Here's how the part is built. I have some questions about the finished solid (model axes, mm). Face numbers are marked on the shaded views. A direction names the side the tool comes from. Coordinates: 2 decimals unless noted, no trailing zeros. Write each loop counter-clockwise with the first axis right and the second up, starting at its lowest first coordinate (ties: lowest second). Pieces come first, ordered by that corner, then holes. Notation, with made-up numbers: (-32, 14) -> (-26, 14) arc R19 ccw to (-26, 43) -> close; hole circle Ø3 at (66, 55). An arc over 180 degrees is marked (long way). Answer in a Markdown table with one row per item. Add a question column.
Autodesk Fusion 360 part; units mm, degrees
sketch "Sketch1" plane through (0, 0, 0) normal (0, 1, 0) x (1, 0, 0)
  line L0 (-6.9583, -4.2531) -> (7.1417, -4.2531)
  line L1 (7.1417, -4.2531) -> (7.1417, 4.7469)
  line L2 (7.1417, 4.7469) -> (-6.9583, 4.7469)
  line L3 (-6.9583, 4.7469) -> (-6.9583, -4.2531)
  line L4 (-6.9583, -4.2531) -> (-2.4583, -4.2531)
  line L5 (-2.4583, -4.2531) -> (-2.4583, 4.7469)
  line L6 (-2.4583, 4.7469) -> (-6.9583, 4.7469)
  line L7 (-6.9583, 4.7469) -> (-6.9583, -4.2531)
  dimension "d4" = 14.1
  dimension "d5" = 9
  dimension "d7" = 4.5
  dimension "d8" = 9
extrude "Extrude1" add sketch "Sketch1" along normal blind 15.4 contours L0 L2 L3 L4 L5 L6 L7
extrude "Extrude2" add sketch "Sketch1" along normal blind 3 contours L0 L1 L2 L5
sketch "Sketch2" plane through (-2.4583, 0, 0) normal (1, 0, 0) x (0, 1, 0)
  line L0 (3, 4.2531) -> (3, -4.7469)
  line L1 (3, -4.7469) -> (15.4, -4.7469)
  line L2 (15.4, -4.7469) -> (15.4, 4.2531)
  line L3 (15.4, 4.2531) -> (3, 4.2531)
  line L4 (3, -0.2469) -> (10.4, -0.2469)
  line L5 (15.4, 4.2531) -> (10.6439, 4.2531)
  line L6 (10.6439, 4.2531) -> (10.6439, -4.7469)
  line L7 (10.6439, -4.7469) -> (15.4, -4.7469)
  line L8 (15.4, -4.7469) -> (15.4, 4.2531)
  dimension "d16" = 7.4
extrude "Extrude3" add sketch "Sketch2" along normal blind 9.6 contours L1 L2 L3 L5 L6 L7 L8
hole "Hole1" at (2.7613, 10.6439, -0.1995) direction (0, 1, 0) diameter 2.529 end through all
fillet "Fillet1" radius 2 1 edges at (-6.9583, 15.4, -0.2469)
fillet "Fillet2" radius 2 1 edges at (-6.9583, 0, -0.2469)
fillet "Fillet3" radius 1 1 edges at (7.1417, 10.6439, -0.2469)
fillet "Fillet4" radius 1 1 edges at (7.1417, 0, -0.2469)
equation "clamp_w = 14.1 mm"
equation "clamp_l = 9 mm"
equation "clamp_bot_thickness = 3 mm"
equation "d4 = clamp_w"
equation "d5 = clamp_l"
equation "clamp_mid_w = 4.5 mm"
equation "d7 = clamp_mid_w"
equation "d8 = clamp_l"
equation "clamp_mid_thickness = wp_gap + clamp_bot_thickness + clamp_top_thickness"
equation "d10 = clamp_mid_thickness"
equation "d12 = clamp_bot_thickness"
equation "clamp_top_thickness = 5 mm"
equation "wp_gap = 7.4 mm"
equation "d16 = wp_gap"
equation "top_clamp_depth = clamp_w - clamp_mid_w"
equation "d18 = top_clamp_depth"
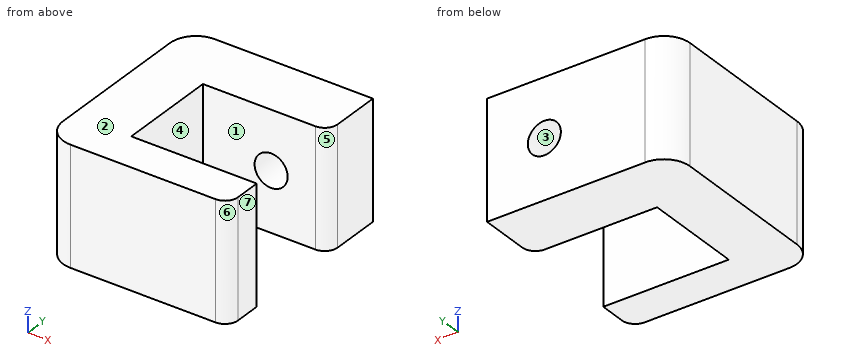
Q1. For the marked faces 1, 2 and 3, which set-ups out of +Z, -Z, +X, -X, +Y, -Y let a thin tool reach every point of the face, with its end or its side?
Q2. I need wall thicknesses on line 1 (Y direction, x = -2, z = 1.25); line 2 (X direction, y = 10.5, z = -1); line 3 (X direction, y = 13.5, z = 2.75). Which ranges of each line are inside material? Lowest first, please. Write a range as [from, to].
Q3. I'm going to push a flat-ended pin straight in: P1, Ø1, axis at x = 3, z = 0, coming from the +Y side. Where does the tip first touch, or does it pass through?
Q4. Imagine slicing it at D-D on x = 3. Please give me the cut outline in (y, z).
Q5. If we mould it in two halves opening along Y, with no side actions, what happens to the marked faces 4, 5, 6 and 7? For each: pulls with the +Y half, pulls with the -Y half, needs draft (parallel to the pull), parting line crosses it, or undercut.
Q6. Imagine slicing it at A-A on x = -2. Please give me the cut outline in (y, z).
Q7. Imagine slicing it at B-B on z = 3. Please give me the cut outline in (x, y), plus the area to 3 significant figures.
Q8. Imagine slicing it at C-C on z = 0.5. Please give me the cut outline in (x, y), plus the area to 3 significant figures.
Result sheet:
| question | item | result |
|---|---|---|
| 1 | face 1 | +Z, -Z, +X |
| 1 | face 2 | +Z, +X, -X, +Y, -Y |
| 1 | face 3 | +Y |
| 2 | line 1 | y = [0, 3], [10.64, 15.4] |
| 2 | line 2 | x = [-6.96, -2.46] |
| 2 | line 3 | x = [-6.96, 7.14] |
| 3 | P1 | stops at y = 3 |
| 4 | outline | (0, -4.75) -> (3, -4.75) -> (3, 4.25) -> (0, 4.25) -> close; (10.64, -4.75) -> (15.4, -4.75) -> (15.4, -1.44) -> (10.64, -1.44) -> close; (10.64, 1.04) -> (15.4, 1.04) -> (15.4, 4.25) -> (10.64, 4.25) -> close |
| 5 | face 4 | undercut |
| 5 | face 5 | undercut |
| 5 | face 6 | pulls with the -Y half |
| 5 | face 7 | needs draft |
| 6 | outline | (0, -4.75) -> (3, -4.75) -> (3, 4.25) -> (0, 4.25) -> close; (10.64, -4.75) -> (15.4, -4.75) -> (15.4, 4.25) -> (10.64, 4.25) -> close |
| 7 | outline | (-6.96, 2) arc R2 ccw to (-4.96, 0) -> (6.14, 0) arc R1 ccw to (7.14, 1) -> (7.14, 3) -> (-2.46, 3) -> (-2.46, 10.64) -> (6.14, 10.64) arc R1 ccw to (7.14, 11.64) -> (7.14, 15.4) -> (-4.96, 15.4) arc R2 ccw to (-6.96, 13.4) -> close |
| 7 | area | 142 mm^2 |
| 8 | outline | (-6.96, 2) arc R2 ccw to (-4.96, 0) -> (6.14, 0) arc R1 ccw to (7.14, 1) -> (7.14, 3) -> (-2.46, 3) -> (-2.46, 10.64) -> (1.71, 10.64) -> (1.71, 15.4) -> (-4.96, 15.4) arc R2 ccw to (-6.96, 13.4) -> close; (3.81, 10.64) -> (6.14, 10.64) arc R1 ccw to (7.14, 11.64) -> (7.14, 15.4) -> (3.81, 15.4) -> close |
| 8 | area | 132 mm^2 |
